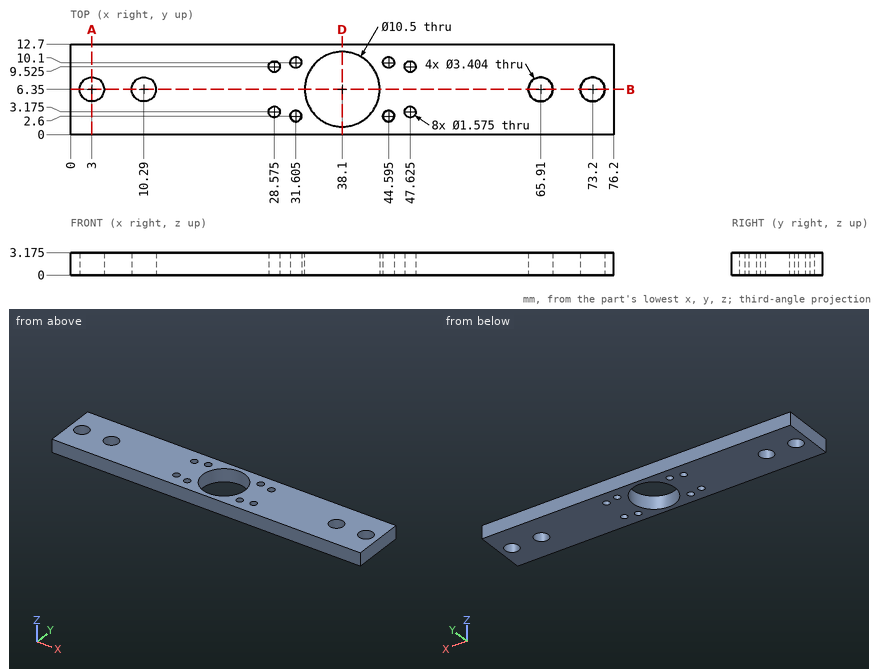
Answer from the drawing. Dimensions are ordinates in mm from the lowest x, y and z of the part. Give positions to 0.01 mm unless a question says otherwise; leave off trailing zeros. Loops run counter-clockwise (first coordinate to the right, second up) from the corner with the lowest first, then second, coordinate; pieces in that order, holes last. Notation, with made-up numbers: (22, 38) - (64, 38) arc R30 cw to (64, 68) - close; hole circle Ø10 at (66, -23.75). An arc over 180 degrees is marked (long way). Answer as CSV lines item,"result". Start each with the question number.
Item 1: A cutting plane is placed at D-D on x = 38.1. Determine the outline of the cut face in (y, z) (1 decimal).
Item 2: Find the intervals of material crossed by line 1 (X direction, y = 6.5, z = 2.2) (1 decimal); line 2 (X direction, y = 2.75, z = 0.35); line 3 (X direction, y = 3.75, z = 0.8) (1 decimal), in increasing order. Write a range as from..to.
Item 3: A cutting plane is placed at B-B on y = 6.35. Count the separate pieces of the cut face and the enclosed holes in it, then the cut area to 3 significant figures.
Item 4: A cutting plane is placed at A-A on x = 3. Determine the outline of the cut face in (y, z) (1 decimal), then the cut area to 3 significant figures.
Found:
1,outline,"(0, 0) - (1.1, 0) - (1.1, 3.2) - (0, 3.2) - close; (11.6, 0) - (12.7, 0) - (12.7, 3.2) - (11.6, 3.2) - close"
2,line 1,"x = 0..1.3, 4.7..8.6, 12..32.9, 43.3..64.2, 67.6..71.5, 74.9..76.2"
2,line 2,"x = 0..27.91, 29.24..30.83, 32.38..34.28, 41.92..43.82, 45.37..46.96, 48.29..76.2"
2,line 3,"x = 0..28, 29.1..33.5, 42.7..47.1, 48.2..76.2"
3,separate pieces,"6"
3,enclosed holes,"0"
3,area,"165 mm^2"
4,outline,"(0, 0) - (4.6, 0) - (4.6, 3.2) - (0, 3.2) - close; (8.1, 0) - (12.7, 0) - (12.7, 3.2) - (8.1, 3.2) - close"
4,area,"29.5 mm^2"
